Here's how the part is built. I have some questions about the finished solid (model axes, mm). Face numbers are marked on the shaded views. A direction names the side the tool comes from. Round coordinates to 2 decimals unless told otherwise and drop trailing zeros. Loops run counter-clockwise (first coordinate to the right, second up) from the corner with the lowest first, then second, coordinate; pieces in that order, holes last. Notation, with made-up numbers: M 1,85.25 L 34,85.25 A12 cw 34,102.25 Z; hole C 42.5,-20 d8. An arc over 180 degrees is marked long. Answer as a JSON object with one key per item and string values.
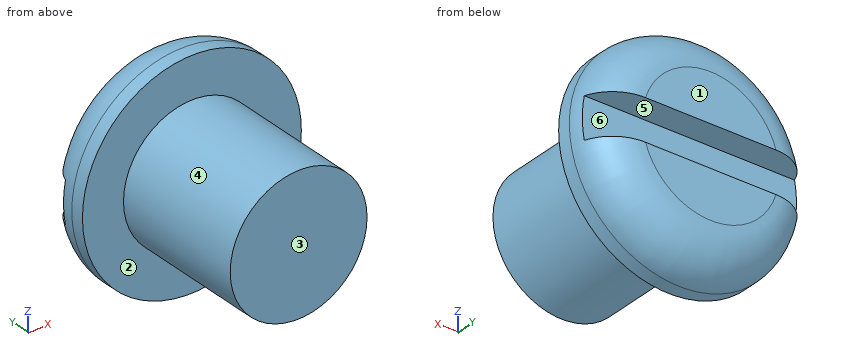
from build123d import *

# Parameters (mm, degrees)
ESBO_O2_W             = 8
ESBO_O2_H             = 1
CORTE_EXTRUS_O1_DEPTH = 0.75


with BuildPart() as part:
    # Esboço1 → Revolução1 (revolve)
    with BuildSketch(Plane.XY):
        with BuildLine():
            Line((0, 0), (2.5, 0))
            Line((2.5, 0), (2.5, 5))
            Line((2.5, 5), (4, 5))
            Line((4, 5), (4, 5.5))
            ThreePointArc((4, 5.5), (3.560660172, 6.560660172), (2.5, 7))
            Line((2.5, 7), (0, 7))
            Line((0, 7), (0, 0))
        make_face()
    revolve(axis=Axis((0, 7, 0), (0, -1, 0)))

    # Esboço2 → Corte-extrusão1 (cut, symmetric)
    with BuildSketch(Plane.XY):
        with Locations((0, 6.5)):
            Rectangle(ESBO_O2_W, ESBO_O2_H)
    extrude(amount=CORTE_EXTRUS_O1_DEPTH, both=True, mode=Mode.SUBTRACT)


solid = part.part
Item 1: I want a section at B-B, the plane z = 0. Please give me the cut outline in (x, y), then the cut area to 3 significant figures.
Resolved:
{"outline": "M -4,5 L -2.5,5 L -2.5,0 L 2.5,0 L 2.5,5 L 4,5 L 4,5.5 A1.5 ccw 3.91,6 L -3.91,6 A1.5 ccw -4,5.5 Z", "area": "33.0 mm²"}
Item 2: I'm going to push flat-ended pins straight in: pin 1 Ø2 at (y, z) = (2.5, 0) entering from -X; pin 2 Ø2.5 at (x, z) = (0.5, -1) entering from -Y; pin 3 Ø0.8 at (x, y) = (-1.5, 6.5) entering from -Z; pin 4 Ø1.5 at (x, y) = (-3, 1) entering from +Z. Where does each tip first touch, or does it pass through?
Resolved:
{"pin 1": "x = -2.5", "pin 2": "y = 0", "pin 3": "z = -3.62", "pin 4": "z = 1.09"}
Item 3: I want a section at D-D, the plane y = 6.5. Please give me the cut outline in (x, z).
Resolved:
{"outline": "M -3.54,-0.75 A3.62 ccw 3.54,-0.75 Z; M -3.54,0.75 L 3.54,0.75 A3.62 ccw Z"}
Item 4: I want a section at C-C, the plane y = 1. Please give me the cut outline in (x, z).
Resolved:
{"outline": "C 0,0 d5"}
Item 5: Please list where these lines run through material, in increasing order: probe 1 along Y at (x, z) = (0, 0); probe 2 along Y at (x, z) = (3.75, 0.25); probe 3 along Z at (x, y) = (-1, 6.75). Write a range as from..to.
Resolved:
{"probe 1": "0..6", "probe 2": "5..6", "probe 3": "-3.18..-0.75, 0.75..3.18"}
Item 6: If we mould it in two halves opening along Z, with no side actions, what happens to the marked faces 3, 4, 5 and 6? For each: pulls with the +Z half, pulls with the -Z half, needs draft (parallel to the pull), parting line crosses it, or undercut.
Resolved:
{"face 3": "needs draft", "face 4": "parting line crosses it", "face 5": "undercut", "face 6": "undercut"}
Item 7: On a 3-axis mill with a long thin cutter (end or side, diameter ignored), from which of +Z, -Z, +X, -X, +Y, -Y can I reach the whole of each face in a straight line? I mean the marked faces 1 and 2. Say none if no direction works.
Resolved:
{"face 1": "+Z, -Z, +X, -X, +Y", "face 2": "-Y"}
Item 8: I want a section at A-A, the plane x = 0. Please give me the cut outline in (y, z).
Resolved:
{"outline": "M 0,-2.5 L 5,-2.5 L 5,-4 L 5.5,-4 A1.5 ccw 7,-2.5 L 7,-0.75 L 6,-0.75 L 6,0.75 L 7,0.75 L 7,2.5 A1.5 ccw 5.5,4 L 5,4 L 5,2.5 L 0,2.5 Z"}
